from build123d import *

# Parameters (mm, degrees)
SKETCH2_W               = 140
SKETCH2_H               = 420
BOSS_EXTRUDE1_DEPTH     = 4
BOSS_EXTRUDE2_DEPTH     = 25
SKETCH4_W               = 10.25
SKETCH4_H               = 80.25
CUT_EXTRUDE1_DEPTH      = 25.4
SKETCH7_W               = 130
SKETCH7_H               = 10
CUT_EXTRUDE2_DEPTH      = 2.45
SKETCH8_W               = 140
SKETCH8_H               = 140
SKETCH8_W_2             = 10.25
SKETCH8_H_2             = 80.25
CUT_EXTRUDE3_DEPTH      = 1
CUT_EXTRUDE3_DEPTH_BACK = 30
SKETCH9_W               = 140
SKETCH9_H               = 10
BOSS_EXTRUDE3_DEPTH     = 2


with BuildPart() as part:
    # Sketch2 → Boss-Extrude1 (new body)
    with BuildSketch(Plane(origin=(0, 0, 0), x_dir=(1, 0, 0), z_dir=(0, 1, 0))):
        Rectangle(SKETCH2_W, SKETCH2_H)
    extrude(amount=BOSS_EXTRUDE1_DEPTH)

    # Sketch3 → Boss-Extrude2 (add)
    with BuildSketch(Plane(origin=(0, 4, 0), x_dir=(1, 0, 0), z_dir=(0, 1, 0))):
        with BuildLine():
            Line((-37.5, -165), (-37.5, -145))
            Line((-37.5, -145), (-43.5, -145))
            Line((-43.5, -145), (-43.5, -165))
            ThreePointArc((-43.5, -165), (0, -208.5), (43.5, -165))
            Line((43.5, -165), (43.5, -145))
            Line((43.5, -145), (37.5, -145))
            Line((37.5, -145), (37.5, -165))
            ThreePointArc((37.5, -165), (0, -202.5), (-37.5, -165))
        make_face()
    extrude(amount=BOSS_EXTRUDE2_DEPTH)

    # Sketch4 → Cut-Extrude1 (cut)
    with BuildSketch(Plane(origin=(0, 4, 0), x_dir=(1, 0, 0), z_dir=(0, 1, 0))):
        with Locations((-59.875, 139.875)):
            Rectangle(SKETCH4_W, SKETCH4_H)
        with Locations((59.875, 139.875)):
            Rectangle(SKETCH4_W, SKETCH4_H)
    extrude(amount=-CUT_EXTRUDE1_DEPTH, mode=Mode.SUBTRACT)

    # Sketch7 → Cut-Extrude2 (cut)
    with BuildSketch(Plane(origin=(0, 4, 0), x_dir=(1, 0, 0), z_dir=(0, 1, 0))):
        with Locations((0, 200)):
            Rectangle(SKETCH7_W, SKETCH7_H)
    extrude(amount=-CUT_EXTRUDE2_DEPTH, mode=Mode.SUBTRACT)

    # Sketch8 → Cut-Extrude3 (cut, two sides)
    with BuildSketch(Plane.XZ) as cut_extrude3_sk:
        with Locations((0, -140)):
            Rectangle(SKETCH8_W, SKETCH8_H)
        with Locations((-59.875, -139.875)):
            Rectangle(SKETCH8_W_2, SKETCH8_H_2, mode=Mode.SUBTRACT)
        with Locations((59.875, -139.875)):
            Rectangle(SKETCH8_W_2, SKETCH8_H_2, mode=Mode.SUBTRACT)
        Rectangle(SKETCH8_W, SKETCH8_H)
    extrude(amount=CUT_EXTRUDE3_DEPTH, mode=Mode.SUBTRACT)
    extrude(cut_extrude3_sk.sketch, amount=-CUT_EXTRUDE3_DEPTH_BACK, mode=Mode.SUBTRACT)

    # Sketch9 → Boss-Extrude3 (add)
    with BuildSketch(Plane.XZ):
        with Locations((0, 65)):
            Rectangle(SKETCH9_W, SKETCH9_H)
    extrude(amount=-BOSS_EXTRUDE3_DEPTH)


solid = part.part
The model under review builds one solid part; all positions refer to its coordinate system, in mm. A direction names the side the tool comes from. Give positions to 0.01 mm unless a question says otherwise; leave off trailing zeros. Order: outer loops, then holes, each group sorted by start corner. A loop starts at its lowest first (then second) coordinate and runs counter-clockwise, first axis right, second up. Notation, with made-up numbers: M -36.5,-39.75 L -32.5,-39.75 A26 ccw -32.5,-24.75 Z; hole C 24.5,-18.5 d5. An arc over 180 degrees is marked long. Answer in a Markdown table with one row per item. Add a question column.
1. Add section A-A on y = 20.25. State the section outline as (x, z) points.
2. For pin 1 Ø10 at (y, z) = (19.5, 156) entering from +X; pin 2 Ø5 at (x, y) = (-41, 21) entering from -Z; pin 3 Ø0.6 at (x, y) = (18, 3) entering from -Z, all flat-tipped, find the tip position at first contact; note any pin that passes through.
3. Add section D-D on x = 0. State the section outline as (y, z) points.
4. Machinability: for faces 5 (the flat face through (-43.5, 16, 155)), 6 (the flat face through (43.5, 16, 155)), 7 (the flat face through (-37.5, 16, 155)), which of the approach directions +Z, -Z, +X, -X, +Y, -Y give a long, thin tool a straight path to every point of the face, cutting with its end or side? Answer none if there is none.
5. Add section B-B on x = -48. State the section outline as (y, z) points, plus the area to 3 significant figures.
6. Mouldability with a two-part tool opening along X and no side actions: class faces 1 (the flat face through (-40, 16, 145)), 2 (the flat face through (70, 2, 134)), 3 (the cylindrical face through (0.82, 16.32, 202.49)), 4 (the flat face through (37.5, 16, 155)) as released by +X, released by -X, zero draft, split by the parting line, or undercut.
7. To check wall thickness, follow line 1 along X through (y, z) = (18.5, 146); line 2 along Y through (x, z) = (19, 147); line 3 along Y through (x, z) = (21, 66). State the ranges of each line that lie inside material, in increasing order.
8. Add section C-C on z = 116.5. State the section outline as (x, y) points, plus the area to 3 significant figures.
The answers:
| question | item | result |
|---|---|---|
| 1 | outline | M -43.5,145 L -37.5,145 L -37.5,165 A37.5 cw 37.5,165 L 37.5,145 L 43.5,145 L 43.5,165 A43.5 ccw -43.5,165 Z |
| 2 | pin 1 | x = 43.5 |
| 2 | pin 2 | z = 145 |
| 2 | pin 3 | z = 70 |
| 3 | outline | M 0,60 L 2,60 L 2,70 L 4,70 L 4,202.5 L 29,202.5 L 29,208.5 L 4,208.5 L 4,210 L 0,210 Z |
| 4 | face 5 | +Z, -Z, -X, +Y |
| 4 | face 6 | +Z, -Z, +X, +Y |
| 4 | face 7 | -Z, +Y |
| 5 | outline | M 0,60 L 2,60 L 2,70 L 4,70 L 4,210 L 0,210 Z |
| 5 | area | 580 mm2 |
| 6 | face 1 | zero draft |
| 6 | face 2 | released by +X |
| 6 | face 3 | undercut |
| 6 | face 4 | undercut |
| 7 | line 1 | -43.5 to -37.5, 37.5 to 43.5 |
| 7 | line 2 | 0 to 4 |
| 7 | line 3 | 0 to 2 |
| 8 | outline | M -70,0 L 70,0 L 70,4 L -70,4 Z |
| 8 | area | 560 mm2 |
